Read the model definition and answer for the solid it produces. Units are mm, in the model's axes. A direction names the side the tool comes from. Round coordinates to 2 decimals unless told otherwise and drop trailing zeros. Loops run counter-clockwise (first coordinate to the right, second up) from the corner with the lowest first, then second, coordinate; pieces in that order, holes last. Notation, with made-up numbers: M 57.25,86.5 L 80.25,86.5 A27 cw 80.25,124.5 Z; hole C 45,-1 d4. An arc over 180 degrees is marked long. Answer as CSV lines item,"result".
```python
from build123d import *

# Parameters (mm, degrees)
SKETCH1_R           = 12
BOSS_EXTRUDE2_DEPTH = 2
SKETCH2_R           = 7.5
BOSS_EXTRUDE3_DEPTH = 12
SKETCH3_R           = 1.35
CUT_EXTRUDE2_DEPTH  = 23
SKETCH4_R           = 1.475
CUT_EXTRUDE4_DEPTH  = 18


with BuildPart() as part:
    # Sketch1 → Boss-Extrude2 (new body)
    with BuildSketch(Plane.XY):
        Circle(SKETCH1_R)
    extrude(amount=BOSS_EXTRUDE2_DEPTH)

    # Sketch2 → Boss-Extrude3 (add)
    with BuildSketch(Plane(origin=(0, 0, 0), x_dir=(-1, 0, 0), z_dir=(0, 0, -1))):
        with Locations((-1.940285, 0.48507125)):
            Circle(SKETCH2_R)
    extrude(amount=BOSS_EXTRUDE3_DEPTH)

    # Sketch3 → Cut-Extrude2 (cut, through all)
    with BuildSketch(Plane.XY.offset(2)):
        with Locations((0, 4)):
            Circle(SKETCH3_R)
        with Locations((0, -4)):
            Circle(SKETCH3_R)
    extrude(amount=-CUT_EXTRUDE2_DEPTH, mode=Mode.SUBTRACT)

    # Sketch4 → Cut-Extrude4 (cut)
    with BuildSketch(Plane.XY.offset(2)):
        with Locations((0, 4)):
            Circle(SKETCH4_R)
        with Locations((0, -4)):
            Circle(SKETCH4_R)
    extrude(amount=-CUT_EXTRUDE4_DEPTH, mode=Mode.SUBTRACT)


solid = part.part
```
1) Determine the mould class of faces 1 (the flat face through (2, 1, -12)), 2 (the cylindrical face through (-11.99, 0.53, 0.99)), 3 (the cylindrical face through (-1.087, 4.997, -4.902)) for opening direction X: released by +X, released by -X, zero draft, split by the parting line, or undercut.
Evaluation:
face 1,"zero draft"
face 2,"split by the parting line"
face 3,"undercut"
2) Find section B-B, the plane x = 0. Give the vertices of the cut face in (y, z) (3 decimals).
Evaluation:
outline,"M -12,0 L -6.76,0 L -6.76,-12 L -5.475,-12 L -5.475,2 L -12,2 Z; M -2.525,-12 L 2.525,-12 L 2.525,2 L -2.525,2 Z; M 5.475,-12 L 7.73,-12 L 7.73,0 L 12,0 L 12,2 L 5.475,2 Z"
3) Each of these flat-tipped pins is pushed along its axis until it touches: P1, Ø1.5, axis at x = -1, z = -1.5, coming from the +Y side; P2, Ø5, axis at y = 7.5, z = -6, coming from the +X side; P3, Ø3, axis at y = -2.5, z = -3.5, coming from the +X side. Where does it stop, or does it pass through?
Evaluation:
P1,"stops at y = 7.66"
P2,"stops at x = 7.93"
P3,"stops at x = 9.29"
4) Find section C-C, the plane x = 3. Give the vertices of the cut face in (y, z), then the cut area to 3 significant figures.
Evaluation:
outline,"M -11.62,0 L -6.94,0 L -6.94,-12 L 7.91,-12 L 7.91,0 L 11.62,0 L 11.62,2 L -11.62,2 Z"
area,"225 mm^2"
5) Find section D-D, the plane y = -1. Give the vertices of the cut face in (x, z).
Evaluation:
outline,"M -11.96,0 L -5.41,0 L -5.41,-12 L 9.29,-12 L 9.29,0 L 11.96,0 L 11.96,2 L -11.96,2 Z"
6) Find section A-A, the plane y = 4. Give the vertices of the cut face in (x, z) (3 decimals).
Evaluation:
outline,"M -11.314,0 L -4.685,0 L -4.685,-12 L -1.475,-12 L -1.475,2 L -11.314,2 Z; M 1.475,-12 L 8.566,-12 L 8.566,0 L 11.314,0 L 11.314,2 L 1.475,2 Z"
7) Straight lines are drawn through the part: line 1 (Y direction, x = 0, z = -6) (3 decimals); line 2 (Z direction, x = -9, y = 2); line 3 (X direction, y = 3.5, z = -2.75). For each, find the intervals that lie inside material, in ascending order.
Evaluation:
line 1,"y = -6.76 to -5.475, -2.525 to 2.525, 5.475 to 7.73"
line 2,"z = 0 to 2"
line 3,"x = -4.93 to -1.39, 1.39 to 8.81"
8) A tool of negligible diameter and unlimited length cuts with its end or side. For faces 4 (the flat face through (-6, -2, 0)), 5 (the cylindrical face through (-0.192, -2.538, -4.902)), from which of +Z, -Z, +X, -X, +Y, -Y can it reach the whole face along a straight path? Write none if from no direction.
Evaluation:
face 4,"-Z"
face 5,"+Z, -Z"
